Work out the finished part from the listing and answer in its coordinate system (mm). A direction names the side the tool comes from. Coordinates: 2 decimals unless noted, no trailing zeros. Loops run counter-clockwise (first coordinate to the right, second up) from the corner with the lowest first, then second, coordinate; pieces in that order, holes last. Notation, with made-up numbers: (65, -25) -> (98, -25) arc R25 cw to (98, 12) -> close; hole circle Ø4 at (20, 41.25). An arc over 180 degrees is marked (long way). Use a Markdown table: item, result.
from build123d import *

# Parameters (mm, degrees)
F0_R     = 1.25
F1_DEPTH = 2.1
F2_W     = 9.4
F2_H     = 4.3
F3_DEPTH = 15
F4_W     = 13
F4_H     = 7.9
F5_DEPTH = 12.9
F6_W     = 13
F6_H     = 7.9
F7_DEPTH = 1.2
F8_W     = 8.6
F8_H     = 3.5
F9_DEPTH = 25
F13_R    = 1
F14_R    = 0.3


with BuildPart() as f1:
    # F0 (on Top) → F1 (new body)
    with BuildSketch(Plane.XY):
        with BuildLine():
            Line((8.560975, 13), (-13.439025, 13))
            ThreePointArc((-13.439025, 13), (-14.853238, 12.414214), (-15.439025, 11))
            Line((-15.439025, 11), (-15.439025, 2))
            ThreePointArc((-15.439025, 2), (-14.853238, 0.585786), (-13.439025, 0))
            Line((-13.439025, 0), (8.560975, 0))
            ThreePointArc((8.560975, 0), (9.975189, 0.585786), (10.560975, 2))
            Line((10.560975, 2), (10.560975, 11))
            ThreePointArc((10.560975, 11), (9.975189, 12.414214), (8.560975, 13))
        make_face()
        with Locations((-12.439025, 6.5)):
            Circle(F0_R, mode=Mode.SUBTRACT)
        with Locations((7.560975, 6.5)):
            Circle(F0_R, mode=Mode.SUBTRACT)
    extrude(amount=F1_DEPTH)


with BuildPart() as f3:
    # F2 (on face) → F3 (new body)
    with BuildSketch(Plane(origin=(0, 0, 0), x_dir=(1, 0, 0), z_dir=(0, 0, -1))):
        with Locations((-2.439025, -6.5)):
            Rectangle(F2_W, F2_H)
    extrude(amount=-F3_DEPTH)


with BuildPart() as f5:
    # F4 (on face) → F5 (new body, through all)
    with BuildSketch(Plane.XY.offset(2.1)):
        with Locations((-2.439025, 6.5)):
            Rectangle(F4_W, F4_H)
    extrude(amount=F5_DEPTH)

    # F11: cut F3
    add(f3.part, mode=Mode.SUBTRACT)


with BuildPart() as f7:
    # F6 (on face) → F7 (new body)
    with BuildSketch(Plane.XY.offset(15)):
        with Locations((-2.439025, 6.5)):
            Rectangle(F6_W, F6_H)
    extrude(amount=F7_DEPTH)


with BuildPart() as f9:
    # F8 (on face) → F9 (new body)
    with BuildSketch(Plane.XY.offset(15)):
        with Locations((-2.439025, 6.5)):
            Rectangle(F8_W, F8_H)
    extrude(amount=F9_DEPTH)


with BuildPart() as f7_1:
    add(f7.part)

    # F10: cut F9
    add(f9.part, mode=Mode.SUBTRACT)


with BuildPart() as f1_1:
    add(f1.part)

    # F11: cut F3
    add(f3.part, mode=Mode.SUBTRACT)


with BuildPart() as f7_2:
    add(f7_1.part)

    # F12: union F5, F1
    add(f5.part)
    add(f1_1.part)

    # F13
    f13_edges = [f7_2.edges().sort_by_distance(p)[0] for p in [
        (-2.439025, 10.45, 2.1),
        (4.060975, 6.5, 2.1),
        (-8.939025, 6.5, 2.1),
        (-2.439025, 2.55, 2.1),
        (-8.939025, 10.45, 9.15),
        (-8.939025, 2.55, 9.15),
        (4.060975, 10.45, 9.15),
        (4.060975, 2.55, 9.15),
        (-8.939025, 6.5, 16.2),
        (-2.439025, 10.45, 16.2),
        (-2.439025, 2.55, 16.2),
        (4.060975, 6.5, 16.2),
    ]]
    fillet(f13_edges, radius=F13_R)

    # F14
    f14_edges = [f7_2.edges().sort_by_distance(p)[0] for p in [
        (2.260975, 6.5, 0),
        (-2.439025, 8.65, 0),
        (-7.139025, 6.5, 0),
        (-2.439025, 4.35, 0),
        (-2.439025, 13, 0),
    ]]
    fillet(f14_edges, radius=F14_R)


solid = f7_2.part
Q1. Consider line 1 (Y direction, x = -2.5, z = 3.75); line 2 (X direction, y = 4.75, z = 9.5); line 3 (Z direction, x = 8.75, y = 4.75). Determine where each line is inside the solid, lowest interval first. Write a range as [from, to].
Solved:
| item | result |
|---|---|
| line 1 | [2.55, 4.35], [8.65, 10.45] |
| line 2 | [-8.94, -7.14], [2.26, 4.06] |
| line 3 | [0, 2.1] |
Q2. Section C-C on z = 8 is taken. Determine the outline of the cut face in (x, y), and give its area (3 significant figures).
Solved:
| item | result |
|---|---|
| outline | (-8.94, 3.55) arc R1 ccw to (-7.94, 2.55) -> (3.06, 2.55) arc R1 ccw to (4.06, 3.55) -> (4.06, 9.45) arc R1 ccw to (3.06, 10.45) -> (-7.94, 10.45) arc R1 ccw to (-8.94, 9.45) -> close; hole (-7.14, 4.35) -> (2.26, 4.35) -> (2.26, 8.65) -> (-7.14, 8.65) -> close |
| area | 61.4 mm² |
Q3. Section B-B on y = 6.5 is taken. State how many separate pieces and enclosed holes the cut face has, and give its area (3 significant figures).
Solved:
| item | result |
|---|---|
| separate pieces | 4 |
| enclosed holes | 0 |
| area | 76.0 mm² |
Q4. Given pin 1 Ø8 at (x, z) = (-8.5, 11.5) entering from -Y; pin 2 Ø5.5 at (x, z) = (-3.5, 7.5) entering from +Y; pin 3 Ø3.5 at (y, z) = (7, 9.5) entering from +X, each flat-ended and moving along its own axis, determine where each tip first touches the part or whether it passes through.
Solved:
| item | result |
|---|---|
| pin 1 | y = 2.55 |
| pin 2 | y = 10.45 |
| pin 3 | x = 4.06 |
Q5. Section D-D on x = 7.5 is taken. Determine the outline of the cut face in (y, z).
Solved:
| item | result |
|---|---|
| outline | (0, 0.3) arc R0.3 ccw to (0.3, 0) -> (5.25, 0) -> (5.25, 2.1) -> (0, 2.1) -> close; (7.75, 0) -> (12.7, 0) arc R0.3 ccw to (13, 0.3) -> (13, 2.1) -> (7.75, 2.1) -> close |
Q6. Section A-A on x = -2.5 is taken. Determine the outline of the cut face in (y, z), and give its area (3 significant figures).
Solved:
| item | result |
|---|---|
| outline | (0, 0.3) arc R0.3 ccw to (0.3, 0) -> (4.05, 0) arc R0.3 ccw to (4.35, 0.3) -> (4.35, 15) -> (4.75, 15) -> (4.75, 16.2) -> (3.55, 16.2) arc R1 ccw to (2.55, 15.2) -> (2.55, 3.1) arc R1 cw to (1.55, 2.1) -> (0, 2.1) -> close; (8.25, 15) -> (8.65, 15) -> (8.65, 0.3) arc R0.3 ccw to (8.95, 0) -> (12.7, 0) arc R0.3 ccw to (13, 0.3) -> (13, 2.1) -> (11.45, 2.1) arc R1 cw to (10.45, 3.1) -> (10.45, 15.2) arc R1 ccw to (9.45, 16.2) -> (8.25, 16.2) -> close |
| area | 69.9 mm² |
Q7. For faces 1 (the flat face through (1.861, 6, 16)), 2 (the flat face through (-3, 10.45, 9)), 3 (the flat face through (-8.939, 6, 9)), determine the directions among +Z, -Z, +X, -X, +Y, -Y from which every point of the face is accessible in a straight line to the end or side of a thin tool.
Solved:
| item | result |
|---|---|
| face 1 | +Z, -Z |
| face 2 | +Z, +X, -X, +Y |
| face 3 | +Z, -X, +Y, -Y |
Q8. Determine the mould class of faces 4 (the cylindrical face through (-2.362, 10.751, 2.385)), 5 (the flat face through (-3, 2.55, 9)), 6 (the flat face through (-3, 8.65, 8)) for opening direction Y: pulls with the +Y half, pulls with the -Y half, needs draft (parallel to the pull), parting line crosses it, or undercut.
Solved:
| item | result |
|---|---|
| face 4 | pulls with the +Y half |
| face 5 | pulls with the -Y half |
| face 6 | undercut |
